from build123d import *

# Parameters (mm, degrees)
BOSS_EXTRUDE1_DEPTH     = 12.5
FILLET1_R               = 12.5
CUT_EXTRUDE1_DEPTH      = 45.370598373
CUT_EXTRUDE1_DEPTH_BACK = 45.370598373
SKETCH2_R               = 2.5
SKETCH3_R               = 2.5
CUT_EXTRUDE2_DEPTH      = 10


with BuildPart() as part:
    # Sketch1 → Boss-Extrude1 (new, symmetric)
    with BuildSketch(Plane(origin=(0, 0, 0), x_dir=(1, 0, 0), z_dir=(0, 1, 0))):
        Polygon((26, -31), (26, 32.5), (27.5, 32.5), (27.5, -32.5), (-27.5, -32.5), (-27.5, 32.5), (-26, 32.5), (-26, -31), align=None)
    extrude(amount=BOSS_EXTRUDE1_DEPTH, both=True)

    # Fillet1
    fillet1_edges = [part.edges().sort_by_distance(p)[0] for p in [
        (-26.75, -12.5, -32.5),
        (-26.75, 12.5, -32.5),
        (26.75, -12.5, -32.5),
        (26.75, 12.5, -32.5),
    ]]
    fillet(fillet1_edges, radius=FILLET1_R - 0.0001)  # a hair under: the kernel refuses the full size

    # Sketch2 → Cut-Extrude1 (cut, two sides: drawn at the far end of the back side and taken through both)
    with BuildSketch(Plane(origin=(0, 0, 0), x_dir=(0, 0, -1), z_dir=(1, 0, 0)).offset(-CUT_EXTRUDE1_DEPTH_BACK)):
        with Locations((20, 0)):
            Circle(SKETCH2_R)
    extrude(amount=CUT_EXTRUDE1_DEPTH + CUT_EXTRUDE1_DEPTH_BACK, mode=Mode.SUBTRACT)

    # Sketch3 → Cut-Extrude2 (cut)
    with BuildSketch(Plane.XY.offset(32.5)):
        Circle(SKETCH3_R)
    extrude(amount=-CUT_EXTRUDE2_DEPTH, mode=Mode.SUBTRACT)


solid = part.part
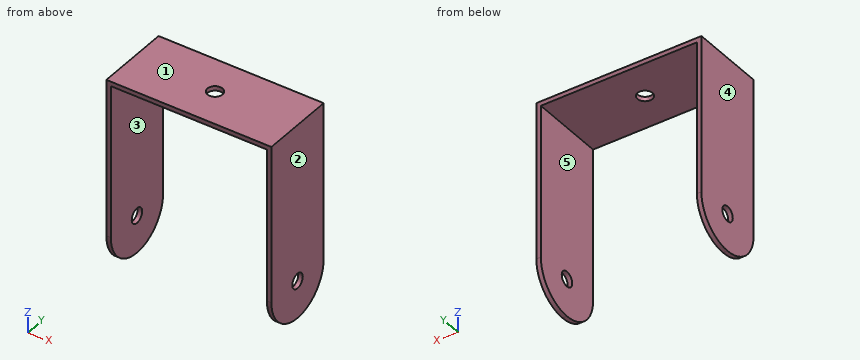
For this review, take the finished solid that the model builds, in its own axes (mm). Face numbers are marked on the shaded views. A direction names the side the tool comes from. Round coordinates to 2 decimals unless told otherwise and drop trailing zeros. Write each loop counter-clockwise with the first axis right and the second up, starting at its lowest first coordinate (ties: lowest second). Pieces come first, ordered by that corner, then holes. Notation, with made-up numbers: (75.25, 35.5) - (105.25, 35.5) arc R18 ccw to (105.25, 56.5) - close; hole circle Ø11 at (-0.5, 60). An arc over 180 degrees is marked (long way). Write item = value, one per line. Start each with the question number.
1. Consider section D-D on y = 4. State the section outline as (x, z) points.
2. Wall thickness on L1, parallel to X at y = -1.5, z = 14; L2, parallel to Y at x = -26.95, z = -20; L3, parallel to Z at x = -26.4, y = 0: over which ranges is each line inside the solid? List them lowest first.
3. For pin 1 Ø6.5 at (y, z) = (0, -20) entering from +X; pin 2 Ø6 at (x, y) = (1.5, 7.5) entering from -Z; pin 3 Ø4 at (x, y) = (0, 0) entering from +Z, all flat-tipped, find the tip position at first contact; note any pin that passes through.
4. Consider section C-C on y = 0.75. State the section outline as (x, z) points.
5. Consider section A-A on z = -10. State the section outline as (x, y) points, plus the area to 3 significant figures.
6. Consider section B-B on x = 0. State the section outline as (y, z) points.
7. For the marked faces 4 and 5, list the 3-axis set-ups (+Z, -Z, +X, -X, +Y, -Y) from which the entire face can be reached by the end or side of a thin tool; tool diameter is ignored.
8. Draft analysis for pull direction X (two halves, no side actions). For the marked faces 1, 2 and 3, state which applies: released by +X, released by -X, zero draft, split by the parting line, or undercut.
Evaluation:
q1.outline = (-27.5, -31.84) - (-26, -31.84) - (-26, 31) - (26, 31) - (26, -31.84) - (27.5, -31.84) - (27.5, 32.5) - (-27.5, 32.5) - close
q2.L1 = -27.5 to -26, 26 to 27.5
q2.L2 = -12.5 to -2.5, 2.5 to 12.5
q2.L3 = -32.5 to -22.5, -17.5 to 32.5
q3.pin_1 = 27.5
q3.pin_2 = 31
q3.pin_3 = through
q4.outline = (-27.5, -32.48) - (-26, -32.48) - (-26, -22.38) - (-27.5, -22.38) - close; (-27.5, -17.62) - (-26, -17.62) - (-26, 31) - (-2.38, 31) - (-2.38, 32.5) - (-27.5, 32.5) - close; (2.38, 31) - (26, 31) - (26, -17.62) - (27.5, -17.62) - (27.5, 32.5) - (2.38, 32.5) - close; (26, -32.48) - (27.5, -32.48) - (27.5, -22.38) - (26, -22.38) - close
q5.outline = (-27.5, -12.5) - (-26, -12.5) - (-26, 12.5) - (-27.5, 12.5) - close; (26, -12.5) - (27.5, -12.5) - (27.5, 12.5) - (26, 12.5) - close
q5.area = 75.0 mm2
q6.outline = (-12.5, 31) - (-2.5, 31) - (-2.5, 32.5) - (-12.5, 32.5) - close; (2.5, 31) - (12.5, 31) - (12.5, 32.5) - (2.5, 32.5) - close
q7.face_4 = +Z, -Z, -X, +Y, -Y
q7.face_5 = -Z, +Y, -Y
q8.face_1 = zero draft
q8.face_2 = released by +X
q8.face_3 = undercut
